```python
from build123d import *

# Parameters (mm, degrees)
SKETCH1_W           = 100
SKETCH1_H           = 26
SKETCH1_R           = 6.1
SKETCH1_R_2         = 4.1
BOSS_EXTRUDE1_DEPTH = 40
SKETCH2_W           = 100
SKETCH2_H           = 26
BOSS_EXTRUDE2_DEPTH = 29.4
CUT_EXTRUDE1_REACH  = 112.797
SKETCH3_W           = 58.5
SKETCH3_H           = 45
SKETCH4_R           = 2.6
CUT_EXTRUDE2_DEPTH  = 111.797111876
CUT_EXTRUDE3_DEPTH  = 4
CUT_EXTRUDE4_START  = -12.2
SKETCH6_W           = 10
SKETCH6_H           = 18
CUT_EXTRUDE4_DEPTH  = 12.2
FILLET1_R           = 5
CUT_EXTRUDE5_DEPTH  = 4
SKETCH8_R           = 2.6
BOSS_EXTRUDE3_DEPTH = 4
SKETCH9_R           = 2.6
BOSS_EXTRUDE4_DEPTH = 4
SKETCH10_R          = 1.5
CUT_EXTRUDE6_DEPTH  = 111.797111876
CUT_EXTRUDE7_DEPTH  = 4
HOLE1_D             = 7.2
HOLE1_DEPTH         = 12.2
HOLE1_CBORE_D       = 10
HOLE1_CBORE_DEPTH   = 8.7


with BuildPart() as part:
    # Sketch1 → Boss-Extrude1 (new body)
    with BuildSketch(Plane.XY):
        with Locations((-50, 13)):
            Rectangle(SKETCH1_W, SKETCH1_H)
        with Locations((-90, 13)):
            Circle(SKETCH1_R, mode=Mode.SUBTRACT)
        with Locations((-66.5, 13)):
            Circle(SKETCH1_R_2, mode=Mode.SUBTRACT)
    boss_extrude1 = extrude(amount=BOSS_EXTRUDE1_DEPTH)

    # Sketch2 → Boss-Extrude2 (add)
    with BuildSketch(Plane(origin=(0, 0, 0), x_dir=(-1, 0, 0), z_dir=(0, 0, -1))):
        with Locations((50, 13)):
            Rectangle(SKETCH2_W, SKETCH2_H)
    boss_extrude2 = extrude(amount=BOSS_EXTRUDE2_DEPTH)

    # Sketch3 → Cut-Extrude1 (cut, up to next)
    with BuildSketch(Plane(origin=(0, 26, 0), x_dir=(1, 0, 0), z_dir=(0, 1, 0)), mode=Mode.PRIVATE) as cut_extrude1_sk1:
        with Locations((-29.25, -5.3)):
            Rectangle(SKETCH3_W, SKETCH3_H)
    cut_extrude1_tool1 = extrude(cut_extrude1_sk1.sketch, amount=-CUT_EXTRUDE1_REACH, mode=Mode.PRIVATE) & part.part
    cut_extrude1 = cut_extrude1_tool1.solids().sort_by_distance((-29.25, 26, 5.3))[0]
    add(cut_extrude1, mode=Mode.SUBTRACT)

    # Mirror2: Boss-Extrude1, Boss-Extrude2, Cut-Extrude1 across plane
    add(boss_extrude1.mirror(Plane(origin=(0, 0, 40), x_dir=(0, 0, 1), z_dir=(-1, 0, 0))))
    add(boss_extrude2.mirror(Plane(origin=(0, 0, 40), x_dir=(0, 0, 1), z_dir=(-1, 0, 0))))
    add(cut_extrude1.mirror(Plane(origin=(0, 0, 40), x_dir=(0, 0, 1), z_dir=(-1, 0, 0))), mode=Mode.SUBTRACT)

    # Sketch4 → Cut-Extrude2 (cut, through all)
    with BuildSketch(Plane(origin=(0, 26, 0), x_dir=(1, 0, 0), z_dir=(0, 1, 0))):
        with Locations(Location((3.5, 23.3, 0), (0, 0, 180))):
            Circle(SKETCH4_R)
        with Locations(Location((29.5, 23.3, 0), (0, 0, 180))):
            Circle(SKETCH4_R)
    cut_extrude2 = extrude(amount=-CUT_EXTRUDE2_DEPTH, mode=Mode.SUBTRACT)

    # Sketch5 → Cut-Extrude3 (cut)
    with BuildSketch(Plane.XZ):
        Polygon((34.234272207, -23.3), (31.867136104, -19.2), (27.132863896, -19.2), (24.765727793, -23.3), (27.132863896, -27.4), (31.867136104, -27.4), align=None)
        Polygon((-1.234272207, -23.3), (1.132863896, -27.4), (5.867136104, -27.4), (8.234272207, -23.3), (5.867136104, -19.2), (1.132863896, -19.2), align=None)
    cut_extrude3 = extrude(amount=-CUT_EXTRUDE3_DEPTH, mode=Mode.SUBTRACT)

    # Mirror3: Cut-Extrude2, Cut-Extrude3 across plane
    add(cut_extrude2.mirror(Plane.XY.offset(5.3)), mode=Mode.SUBTRACT)
    add(cut_extrude3.mirror(Plane.XY.offset(5.3)), mode=Mode.SUBTRACT)

    # Sketch6 → Cut-Extrude4 (cut)
    with BuildSketch(Plane.XY.offset(40).offset(CUT_EXTRUDE4_START)):
        with Locations((-23.2, 13)):
            Rectangle(SKETCH6_W, SKETCH6_H)
    extrude(amount=CUT_EXTRUDE4_DEPTH, mode=Mode.SUBTRACT)

    # Fillet1
    fillet1_edges = [part.edges().sort_by_distance(p)[0] for p in [
        (-58.5, 26, 5.3),
        (-58.5, 0, 5.3),
        (100, 0, 5.3),
        (100, 26, 5.3),
        (-100, 0, 5.3),
        (-100, 26, 5.3),
        (58.5, 0, 5.3),
        (58.5, 26, 5.3),
    ]]
    fillet(fillet1_edges, radius=FILLET1_R)

    # Sketch7 → Cut-Extrude5 (cut)
    with BuildSketch(Plane(origin=(0, 26, 0), x_dir=(1, 0, 0), z_dir=(0, 1, 0))):
        Polygon((8.349742261, 23.3), (5.924871131, 27.5), (1.075128869, 27.5), (-1.349742261, 23.3), (1.075128869, 19.1), (5.924871131, 19.1), align=None)
        Polygon((34.349742261, 23.3), (31.924871131, 27.5), (27.075128869, 27.5), (24.650257739, 23.3), (27.075128869, 19.1), (31.924871131, 19.1), align=None)
    cut_extrude5 = extrude(amount=-CUT_EXTRUDE5_DEPTH, mode=Mode.SUBTRACT)

    # Mirror4: Cut-Extrude5 across plane
    add(cut_extrude5.mirror(Plane.XY.offset(5.3)), mode=Mode.SUBTRACT)

    # Sketch8 → Boss-Extrude3 (add)
    # profile 1 of 2: a face of its own
    with BuildSketch(Plane.XZ.offset(-4)):
        Polygon((27.132863896, 38), (31.867136104, 38), (34.234272207, 33.9), (31.867136104, 29.8), (27.132863896, 29.8), (24.765727793, 33.9), align=None)
        with Locations(Location((29.5, 33.9, 0), (0, 0, 180))):
            Circle(SKETCH8_R, mode=Mode.SUBTRACT)
    # profile 2 of 2: a face of its own
    with BuildSketch(Plane.XZ.offset(-4)):
        Polygon((1.132863896, 38), (5.867136104, 38), (8.234272207, 33.9), (5.867136104, 29.8), (1.132863896, 29.8), (-1.234272207, 33.9), align=None)
        with Locations(Location((3.5, 33.9, 0), (0, 0, 180))):
            Circle(SKETCH8_R, mode=Mode.SUBTRACT)
    extrude(amount=BOSS_EXTRUDE3_DEPTH)

    # Sketch9 → Boss-Extrude4 (add)
    # profile 1 of 2: a face of its own
    with BuildSketch(Plane.XZ.offset(-4)):
        Polygon((31.867136104, -19.2), (27.132863896, -19.2), (24.765727793, -23.3), (27.132863896, -27.4), (31.867136104, -27.4), (34.234272207, -23.3), align=None)
        with Locations(Location((29.5, -23.3, 0), (0, 0, 180))):
            Circle(SKETCH9_R, mode=Mode.SUBTRACT)
    # profile 2 of 2: a face of its own
    with BuildSketch(Plane.XZ.offset(-4)):
        Polygon((1.132863896, -19.2), (-1.234272207, -23.3), (1.132863896, -27.4), (5.867136104, -27.4), (8.234272207, -23.3), (5.867136104, -19.2), align=None)
        with Locations(Location((3.5, -23.3, 0), (0, 0, 180))):
            Circle(SKETCH9_R, mode=Mode.SUBTRACT)
    extrude(amount=BOSS_EXTRUDE4_DEPTH)

    # Sketch10 → Cut-Extrude6 (cut, through all)
    with BuildSketch(Plane.XZ):
        with Locations(Location((-90, 10, 0), (0, 0, 270))):
            Circle(SKETCH10_R)
        with Locations(Location((90, 10, 0), (0, 0, 270))):
            Circle(SKETCH10_R)
    extrude(amount=-CUT_EXTRUDE6_DEPTH, mode=Mode.SUBTRACT)

    # Sketch11 → Cut-Extrude7 (cut)
    with BuildSketch(Plane(origin=(0, 26, 0), x_dir=(1, 0, 0), z_dir=(0, 1, 0))):
        Polygon((-90, -13.175426481), (-87.25, -11.58771324), (-87.25, -8.41228676), (-90, -6.824573519), (-92.75, -8.41228676), (-92.75, -11.58771324), align=None)
        Polygon((90, -13.175426481), (92.75, -11.58771324), (92.75, -8.41228676), (90, -6.824573519), (87.25, -8.41228676), (87.25, -11.58771324), align=None)
    extrude(amount=-CUT_EXTRUDE7_DEPTH, mode=Mode.SUBTRACT)

    # Hole1
    with Locations(Plane(origin=(-52.21, 7.5, 27.8), x_dir=(-1, 0, 0), z_dir=(0, 0, -1))):
        with Locations((0, 0)):
            CounterBoreHole(HOLE1_D / 2, HOLE1_CBORE_D / 2, HOLE1_CBORE_DEPTH, depth=HOLE1_DEPTH)


solid = part.part
```
Geometry: final body of the model. Coordinates: model frame, mm. A direction names the side the tool comes from. Round coordinates to 2 decimals unless told otherwise and drop trailing zeros. Order: outer loops, then holes, each group sorted by start corner. A loop starts at its lowest first (then second) coordinate and runs counter-clockwise, first axis right, second up. Notation, with made-up numbers: M -5.5,-28.75 L -0.5,-28.75 A24 ccw -0.5,1.25 Z; hole C -2,38.25 d1. An arc over 180 degrees is marked long. Use one line per item in the form item = value. Start each with the question number.
Q1. Material intervals for line 1 (X direction, y = 21.35, z = 10); line 2 (Z direction, x = 55, y = 23.5); line 3 (Z direction, x = -91, y = 3.5), sorted ascending. Write a range as [from, to].
Q2. Cut plane C-C (z = -3.5). Return loops of the section in (x, y).
Q3. Cut plane D-D (x = 29.5). Return loops of the section in (y, z).
Q4. Pin query (flat end, axial travel): pin 1 Ø2.5 at (x, z) = (4.5, 35.5) entering from +Y; pin 2 Ø3.5 at (x, y) = (91, 13) entering from +Z; pin 3 Ø3 at (x, z) = (3.5, 33.9) entering from +Y; pin 4 Ø1 at (y, z) = (23.5, 9.5) entering from +X. Return the tip coordinate at first contact, or that it passes through.
Q5. Access query for faces 3 (the face through (-23, 22, 34)), 4 (the face through (-91.3, 22, 11.4)), 5 (the face through (32.1, 11.2, 33.8)), 6 (the face through (-47.215, 7.72, 32.089)), 7 (the face through (59.93, 1.5, 5.62)). Directions: +Z, -Z, +X, -X, +Y, -Y. A direction counts if a zero-diameter tool reaches every point of the face in a straight line with its end or side. Return the directions, or none.
Q6. Mould query, pull axis X, two halves, no side actions, for faces 1 (the face through (1, 13, 40)), 2 (the face through (32, 22, 36)). Classes: +X half, -X half, draft (parallel to the pull), parting line (faces both ways), or undercut.
Q7. Cut plane B-B (x = -35.5). Return loops of the section in (y, z), and give its area (3 significant figures).
Q8. Cut plane A-A (z = 16.5). Return loops of the section in (x, y).
Geometry results:
q1.line_1 = [-99.99, -91.5], [-88.5, -58.51], [58.51, 88.5], [91.5, 99.99]
q1.line_2 = [-29.4, -17.2], [27.8, 40]
q1.line_3 = [-29.4, 8.88], [11.12, 40]
q2.outline = M -100,5 A5 ccw -95,0 L -63.5,0 A5 ccw -58.5,5 L -58.5,21 A5 ccw -63.5,26 L -95,26 A5 ccw -100,21 Z; M 58.5,5 A5 ccw 63.5,0 L 95,0 A5 ccw 100,5 L 100,21 A5 ccw 95,26 L 63.5,26 A5 ccw 58.5,21 Z
q3.outline = M 0,-29.4 L 26,-29.4 L 26,-27.5 L 22,-27.5 L 22,-25.9 L 0,-25.9 Z; M 0,-20.7 L 22,-20.7 L 22,-19.1 L 26,-19.1 L 26,-17.2 L 0,-17.2 Z; M 0,27.8 L 26,27.8 L 26,29.7 L 22,29.7 L 22,31.3 L 0,31.3 Z; M 0,36.5 L 22,36.5 L 22,38.1 L 26,38.1 L 26,40 L 0,40 Z
q4.pin_1 = 22
q4.pin_2 = 0
q4.pin_3 = through
q4.pin_4 = 99.58
q5.face_3 = +Z
q5.face_4 = +Y
q5.face_5 = +Y, -Y
q5.face_6 = none
q5.face_7 = -Y
q6.face_1 = draft
q6.face_2 = undercut
q7.outline = M 0,-29.4 L 26,-29.4 L 26,-17.2 L 0,-17.2 Z; M 0,27.8 L 26,27.8 L 26,40 L 0,40 Z
q7.area = 634 mm^2
q8.outline = M -100,5 A5 ccw -95,0 L -63.5,0 A5 ccw -58.5,5 L -58.5,21 A5 ccw -63.5,26 L -95,26 A5 ccw -100,21 Z; M 58.5,5 A5 ccw 63.5,0 L 95,0 A5 ccw 100,5 L 100,21 A5 ccw 95,26 L 63.5,26 A5 ccw 58.5,21 Z; hole C -90,13 d12.2; hole C -66.5,13 d8.2; hole C 66.5,13 d8.2; hole C 90,13 d12.2
